Read the model definition and answer for the solid it produces. Units are mm, in the model's axes. A direction names the side the tool comes from. Give positions to 0.01 mm unless a question says otherwise; leave off trailing zeros. Order: outer loops, then holes, each group sorted by start corner. A loop starts at its lowest first (then second) coordinate and runs counter-clockwise, first axis right, second up. Notation, with made-up numbers: (-32.5, -10) -> (-12.5, -10) arc R27 cw to (-12.5, 11) -> close; hole circle Ø9 at (69, -31). An arc over 180 degrees is marked (long way). One line per question, with ' | ' between items. Start each with the question number.
```python
from build123d import *

# Parameters (mm, degrees)
BOSS_EXTRU_1_DEPTH      = 20
ESQUISSE2_R             = 3
ENL_V_MAT_EXTRU_1_DEPTH = 4.5
ESQUISSE3_R             = 1.75
ENL_V_MAT_EXTRU_2_DEPTH = 21.988091862


with BuildPart() as part:
    # Esquisse1 → Boss.-Extru.1 (new body)
    with BuildSketch(Plane.XY):
        Polygon((-4.5, 0), (4.5, 0), (4.5, 3.5), (3.5, 4), (3.5, 4.5), (4.5, 5), (4.5, 5.5), (-4.5, 5.5), (-4.5, 5), (-3.5, 4.5), (-3.5, 4), (-4.5, 3.5), align=None)
    extrude(amount=BOSS_EXTRU_1_DEPTH)

    # Esquisse2 → Enlèv. mat.-Extru.1 (cut)
    with BuildSketch(Plane(origin=(0, 5.5, 0), x_dir=(1, 0, 0), z_dir=(0, 1, 0))):
        with Locations(Location((0, -10, 0), (0, 0, 180))):
            Circle(ESQUISSE2_R)
    extrude(amount=-ENL_V_MAT_EXTRU_1_DEPTH, mode=Mode.SUBTRACT)

    # Esquisse3 → Enlèv. mat.-Extru.2 (cut, through all)
    with BuildSketch(Plane(origin=(0, 1, 0), x_dir=(1, 0, 0), z_dir=(0, 1, 0))):
        with Locations(Location((0, -10, 0), (0, 0, 180))):
            Circle(ESQUISSE3_R)
    extrude(amount=-ENL_V_MAT_EXTRU_2_DEPTH, mode=Mode.SUBTRACT)


solid = part.part
```
Q1. A cutting plane is placed at D-D, the plane x = 4. Determine the outline of the cut face in (y, z), then the cut area to 3 significant figures.
Q2. A cutting plane is placed at B-B, the plane x = 0. Determine the outline of the cut face in (y, z).
Q3. A cutting plane is placed at A-A, the plane z = 10. Determine the outline of the cut face in (x, y), then the cut area to 3 significant figures.
Q4. A cutting plane is placed at C-C, the plane y = 4.2. Determine the outline of the cut face in (x, z).
Q5. Given P1, Ø2, axis at x = -1, y = 4.5, coming from the -Z side, flat-ended and moving along its own axis, determine where the tip first touches the part or whether it passes through.
Q6. Determine the mould class of faces 5 (the flat face through (3.993, 4.746, 9.86)), 6 (the cylindrical face through (0.228, 0.507, 11.735)), 7 (the flat face through (0, 3, 20)) for opening direction Z: pulls with the +Z half, pulls with the -Z half, needs draft (parallel to the pull), parting line crosses it, or undercut.
Q7. Which of the six approach directions +Z, -Z, +X, -X, +Y, -Y give full straight-line access (tool end or side, diameter ignored) to faces 1 (the flat face through (-4.5, 2, 10)), 2 (the cylindrical face through (-2.86, 3.28, 10.9)), 3 (the flat face through (4.007, 3.746, 9.86)), 4 (the flat face through (-3.993, 3.754, 9.86))?
Q8. Find the intervals of material crossed by line 1 (Z direction, x = 0, y = 2.65); line 2 (Z direction, x = -1.5, y = 3.85); line 3 (Y direction, x = -1.5, z = 7.5), in increasing order.
Geometry results:
1) outline: (0, 0) -> (3.75, 0) -> (3.75, 20) -> (0, 20) -> close; (4.75, 0) -> (5.5, 0) -> (5.5, 20) -> (4.75, 20) -> close | area: 90.0 mm²
2) outline: (0, 0) -> (5.5, 0) -> (5.5, 7) -> (1, 7) -> (1, 8.25) -> (0, 8.25) -> close; (0, 11.75) -> (1, 11.75) -> (1, 13) -> (5.5, 13) -> (5.5, 20) -> (0, 20) -> close
3) outline: (-4.5, 0) -> (-1.75, 0) -> (-1.75, 1) -> (-3, 1) -> (-3, 5.5) -> (-4.5, 5.5) -> (-4.5, 5) -> (-3.5, 4.5) -> (-3.5, 4) -> (-4.5, 3.5) -> close; (1.75, 0) -> (4.5, 0) -> (4.5, 3.5) -> (3.5, 4) -> (3.5, 4.5) -> (4.5, 5) -> (4.5, 5.5) -> (3, 5.5) -> (3, 1) -> (1.75, 1) -> close | area: 17.0 mm²
4) outline: (-3.5, 0) -> (3.5, 0) -> (3.5, 20) -> (-3.5, 20) -> close; hole circle Ø6 at (0, 10)
5) P1: z = 0
6) face 5: needs draft | face 6: undercut | face 7: pulls with the +Z half
7) face 1: +Z, -Z, -X, +Y, -Y | face 2: +Y | face 3: +Z, -Z, +X | face 4: +Z, -Z, -X
8) line 1: 0 to 7, 13 to 20 | line 2: 0 to 7.4, 12.6 to 20 | line 3: 0 to 1
